Verification items for the finished model (mm, model axes). A direction names the side the tool comes from. Round coordinates to 2 decimals unless told otherwise and drop trailing zeros. Write each loop counter-clockwise with the first axis right and the second up, starting at its lowest first coordinate (ties: lowest second). Pieces come first, ordered by that corner, then holes. Notation, with made-up numbers: M -34.5,-8.75 L 6.5,-8.75 A25 ccw 6.5,5.25 Z; hole C -33.5,26.5 d6. An arc over 180 degrees is marked long. One line per item, written item: value. Start each with the question number.
Item 1: Section check D-D, the plane y = -27. Record the cut outline in (x, z), then the cut area to 3 significant figures.
Item 2: Section check B-B, the plane z = 0. Record the cut outline in (x, y), then the cut area to 3 significant figures.
Item 3: Draft check along Y on faces 1 (the face through (2.96, 17.95, -7.67)), 2 (the face through (3, -35.29, 18)), 3 (the face through (2.96, -8.7, -18.18)), 4 (the face through (6, -19, -2)). Enter one of: +Y half, -Y half, draft (parallel to the pull), parting line (faces both ways), or undercut.
Item 4: Tool access check on faces 5 (the face through (10, -23, 0)), 6 (the face through (3, -35.29, -18)), 7 (the face through (4, -11.4, 14.8)), 8 (the face through (0, -15, -5)), 9 (the face through (2.958, -18.326, -7.019)). Record the directions out of +Z, -Z, +X, -X, +Y, -Y that give a thin tool (end or side, any length) a straight path to the whole face; none if there is none.
Item 5: Section check A-A, the plane y = 0. Record the cut outline in (x, z), then the cut area to 3 significant figures.
Item 6: Gauge pin test, flat ends, axial feed: pin 1 (1.8 mm diameter, centred on x = 10, z = -17, fed in from -Y); pin 2 (10 mm diameter, centred on y = 11.5, z = -6.5, fed in from -X); pin 3 (18.5 mm diameter, centred on y = -2, z = 9, fed in from +X); pin 4 (2 mm diameter, centred on x = 3.46, z = -17.5, fed in from +Y). Record the tip position at first contact, or that the pin passes through.
Item 7: Thickness scan on probe 1 along X at (y, z) = (-37, -17); probe 2 along Z at (x, y) = (1.5, 0.5); probe 3 along Z at (x, y) = (13.25, -19). Record the ranges inside material, lowest first. Write a range as from..to.
Item 8: Section check C-C, the plane x = 7.5. Record the cut outline in (y, z), then the cut area to 3 significant figures.
from build123d import *

# Parameters (mm, degrees)
SKETCH_1_R               = 18.68
SKETCH_1_R_2             = 15.652173913
EXTRUDE_2_DEPTH          = 2
SKETCH_1_4_R             = 23
SKETCH_1_4_R_2           = 1.25
SKETCH_1_4_R_3           = 18.68
EXTRUDE_3_DEPTH          = 6
EXTRUDE_4_DEPTH          = 14
SKETCH_4_R               = 1.8
CUT_EXTRUDE_1_DEPTH      = 5
MIRROR_2_COPY_1_SKETCH_R = 1.8
MIRROR_2_COPY_1_DEPTH    = 5


with BuildPart() as part:
    # Sketch 1 → Extrude 2 (new body)
    with BuildSketch(Plane(origin=(0, 0, 0), x_dir=(0, 0, -1), z_dir=(1, 0, 0))):
        Circle(SKETCH_1_R)
        Circle(SKETCH_1_R_2, mode=Mode.SUBTRACT)
    extrude(amount=EXTRUDE_2_DEPTH)



with BuildPart() as body_2:
    # Sketch 1_4 → Extrude 3 (new body)
    with BuildSketch(Plane(origin=(0, 0, 0), x_dir=(0, 0, -1), z_dir=(1, 0, 0))):
        Circle(SKETCH_1_4_R)
        with Locations((-7.940681222, 19.1705003)):
            Circle(SKETCH_1_4_R_2, mode=Mode.SUBTRACT)
        with Locations((-19.1705003, 7.940681222)):
            Circle(SKETCH_1_4_R_2, mode=Mode.SUBTRACT)
        with Locations((-19.1705003, -7.940681222)):
            Circle(SKETCH_1_4_R_2, mode=Mode.SUBTRACT)
        with Locations((-7.940681222, -19.1705003)):
            Circle(SKETCH_1_4_R_2, mode=Mode.SUBTRACT)
        with Locations((7.940681222, -19.1705003)):
            Circle(SKETCH_1_4_R_2, mode=Mode.SUBTRACT)
        with Locations((19.1705003, -7.940681222)):
            Circle(SKETCH_1_4_R_2, mode=Mode.SUBTRACT)
        with Locations((19.1705003, 7.940681222)):
            Circle(SKETCH_1_4_R_2, mode=Mode.SUBTRACT)
        with Locations((7.940681222, 19.1705003)):
            Circle(SKETCH_1_4_R_2, mode=Mode.SUBTRACT)
        Circle(SKETCH_1_4_R_3, mode=Mode.SUBTRACT)
    extrude(amount=EXTRUDE_3_DEPTH)


with BuildPart() as part_1:
    add(part.part)

    add(body_2.part)  # Extrude 4 merges body 2
    # Sketch 2 → Extrude 4 (add)
    with BuildSketch(Plane.ZY):
        with BuildLine():
            Line((-21.5, -40.29), (21.5, -40.29))
            Line((21.5, -40.29), (21.5, -8.170067319))
            ThreePointArc((21.5, -8.170067319), (0, -23), (-21.5, -8.170067319))
            Line((-21.5, -8.170067319), (-21.5, -40.29))
        make_face()
    extrude(amount=-EXTRUDE_4_DEPTH)

    # Sketch 4 → Cut-Extrude 1 (cut)
    with BuildSketch(Plane(origin=(0, -40.29, 0), x_dir=(-1, 0, 0), z_dir=(0, -1, 0))):
        with Locations(Location((-10.536326609, -17.5, 0), (0, 0, 90))):
            Circle(SKETCH_4_R)
    cut_extrude_1 = extrude(amount=-CUT_EXTRUDE_1_DEPTH, mode=Mode.SUBTRACT)

    # Mirror 1: Cut-Extrude 1 across plane
    add(cut_extrude_1.mirror(Plane.XY), mode=Mode.SUBTRACT)

    # Mirror 2: Cut-Extrude 1 across plane
    add(cut_extrude_1.mirror(Plane.ZY.offset(-7)), mode=Mode.SUBTRACT)

    # Mirror 2 copy 1 sketch → Mirror 2 copy 1 (cut)
    with BuildSketch(Plane(origin=(14, -40.29, 0), x_dir=(1, 0, 0), z_dir=(0, -1, 0))):
        with Locations(Location((-10.536326609, -17.5, 0), (0, 0, 90))):
            Circle(MIRROR_2_COPY_1_SKETCH_R)
    extrude(amount=-MIRROR_2_COPY_1_DEPTH, mode=Mode.SUBTRACT)


solid = part_1.part
Response values:
1. outline: M 0,-21.5 L 14,-21.5 L 14,21.5 L 0,21.5 Z
1. area: 602 mm2
2. outline: M 0,-40.29 L 14,-40.29 L 14,-23 L 6,-23 L 6,-18.68 L 2,-18.68 L 2,-15.65 L 0,-15.65 Z; M 0,15.65 L 2,15.65 L 2,18.68 L 6,18.68 L 6,23 L 0,23 Z
2. area: 306 mm2
3. face 1: undercut
3. face 2: -Y half
3. face 3: undercut
3. face 4: draft
4. face 5: +X, +Y
4. face 6: -Y
4. face 7: +X
4. face 8: +Z, -Z, -X, +Y, -Y
4. face 9: +X, -X
5. outline: M 0,-23 L 6,-23 L 6,-18.68 L 2,-18.68 L 2,-15.65 L 0,-15.65 Z; M 0,15.65 L 2,15.65 L 2,18.68 L 6,18.68 L 6,23 L 0,23 Z
5. area: 64.0 mm2
6. pin 1: stops at y = -35.29
6. pin 2: stops at x = 0
6. pin 3: stops at x = 2
6. pin 4: stops at y = 16.02
7. probe 1: x = 0..1.73, 5.19..8.81, 12.27..14
7. probe 2: z = -22.99..-15.64, 15.64..22.99
7. probe 3: z = -21.5..-12.96, 12.96..21.5
8. outline: M -40.29,-21.5 L -8.17,-21.5 A23 cw -8.17,21.5 L -40.29,21.5 Z
8. area: 918 mm2
